```python
from build123d import *
from OCP.BRepFilletAPI import BRepFilletAPI_MakeChamfer

# Parameters (mm, degrees)
SKETCH_1_W           = 177
SKETCH_1_H           = 15
EXTRUDE_1_DEPTH      = 5
SKETCH_3_W           = 15
SKETCH_3_H           = 55
EXTRUDE_3_DEPTH      = 5
SKETCH_9_W           = 33
SKETCH_9_H           = 35
EXTRUDE_5_DEPTH      = 5
CUT_EXTRUDE_4_REACH  = 115.989
CUT_EXTRUDE_5_REACH  = 115.989
SKETCH_10_R          = 3
SKETCH_13_W          = 28
SKETCH_13_H          = 25
CUT_EXTRUDE_8_DEPTH  = 10
CHAMFER_4_SIZE       = 5
FILLET_3_R           = 3
SKETCH_14_W          = 6
SKETCH_14_H          = 11
CUT_EXTRUDE_9_DEPTH  = 10
SKETCH_15_R          = 3.5
CUT_EXTRUDE_10_DEPTH = 10
CHAMFER_5_SIZE       = 2
CHAMFER_5_SIZE2      = 2.22122503


with BuildPart() as part:
    # 스케치1 → 보스-돌출1 (new body)
    with BuildSketch(Plane.XY):
        Rectangle(SKETCH_1_W, SKETCH_1_H)
    extrude(amount=EXTRUDE_1_DEPTH)

    # 스케치3 → 보스-돌출3 (add)
    with BuildSketch(Plane.XY.offset(5)):
        with Locations((96, -20)):
            Rectangle(SKETCH_3_W, SKETCH_3_H)
        with Locations((-96, -20)):
            Rectangle(SKETCH_3_W, SKETCH_3_H)
    extrude(amount=-EXTRUDE_3_DEPTH)

    # 스케치9 → 보스-돌출5 (add)
    with BuildSketch(Plane.XY.offset(5)):
        with Locations((-72, -30)):
            Rectangle(SKETCH_9_W, SKETCH_9_H)
        with Locations((72, -30)):
            Rectangle(SKETCH_9_W, SKETCH_9_H)
    extrude(amount=-EXTRUDE_5_DEPTH)

    # 스케치8 → 컷-돌출4 (cut, up to next)
    with BuildSketch(Plane.XY.offset(5), mode=Mode.PRIVATE) as cut_extrude_4_sk1:
        with BuildLine():
            Line((-88.5, -7.5), (-88.7, -7.5))
            ThreePointArc((-88.7, -7.5), (-89.407106781, -7.792893219), (-89.7, -8.5))
            Line((-89.7, -8.5), (-89.7, -11.5))
            ThreePointArc((-89.7, -11.5), (-89.407106781, -12.207106781), (-88.7, -12.5))
            Line((-88.7, -12.5), (-88.5, -12.5))
            Line((-88.5, -12.5), (-88.5, -7.5))
        make_face()
    cut_extrude_4_tool1 = extrude(cut_extrude_4_sk1.sketch, amount=-CUT_EXTRUDE_4_REACH, mode=Mode.PRIVATE) & part.part
    # 스케치8 → 컷-돌출4 (cut, up to next)
    with BuildSketch(Plane.XY.offset(5), mode=Mode.PRIVATE) as cut_extrude_4_sk2:
        with BuildLine():
            Line((88.5, -7.5), (88.7, -7.5))
            ThreePointArc((88.7, -7.5), (89.407106781, -7.792893219), (89.7, -8.5))
            Line((89.7, -8.5), (89.7, -11.5))
            ThreePointArc((89.7, -11.5), (89.407106781, -12.207106781), (88.7, -12.5))
            Line((88.7, -12.5), (88.5, -12.5))
            Line((88.5, -12.5), (88.5, -7.5))
        make_face()
    cut_extrude_4_tool2 = extrude(cut_extrude_4_sk2.sketch, amount=-CUT_EXTRUDE_4_REACH, mode=Mode.PRIVATE) & part.part
    add(cut_extrude_4_tool1.solids().sort_by_distance((-89.070982, -10, 5))[0], mode=Mode.SUBTRACT)
    add(cut_extrude_4_tool2.solids().sort_by_distance((89.070982, -10, 5))[0], mode=Mode.SUBTRACT)

    # 스케치10 → 컷-돌출5 (cut, up to next)
    with BuildSketch(Plane.XY.offset(5), mode=Mode.PRIVATE) as cut_extrude_5_sk1:
        with Locations((65, -36.5)):
            Circle(SKETCH_10_R)
    cut_extrude_5_tool1 = extrude(cut_extrude_5_sk1.sketch, amount=-CUT_EXTRUDE_5_REACH, mode=Mode.PRIVATE) & part.part
    # 스케치10 → 컷-돌출5 (cut, up to next)
    with BuildSketch(Plane.XY.offset(5), mode=Mode.PRIVATE) as cut_extrude_5_sk2:
        with Locations((-65, -36.5)):
            Circle(SKETCH_10_R)
    cut_extrude_5_tool2 = extrude(cut_extrude_5_sk2.sketch, amount=-CUT_EXTRUDE_5_REACH, mode=Mode.PRIVATE) & part.part
    add(cut_extrude_5_tool1.solids().sort_by_distance((65, -36.5, 5))[0], mode=Mode.SUBTRACT)
    add(cut_extrude_5_tool2.solids().sort_by_distance((-65, -36.5, 5))[0], mode=Mode.SUBTRACT)

    # 스케치13 → 컷-돌출8 (cut)
    with BuildSketch(Plane(origin=(0, 0, 0), x_dir=(-1, 0, 0), z_dir=(0, 0, -1))):
        with Locations((-89.5, -35)):
            Rectangle(SKETCH_13_W, SKETCH_13_H)
        with Locations((89.5, -35)):
            Rectangle(SKETCH_13_W, SKETCH_13_H)
    extrude(amount=-CUT_EXTRUDE_8_DEPTH, mode=Mode.SUBTRACT)

    # 모따기4
    chamfer_4_edges = [part.edges().sort_by_distance(p)[0] for p in [
        (103.5, -22.5, 2.5),
        (-103.5, -22.5, 2.5),
        (103.5, 7.5, 2.5),
        (-103.5, 7.5, 2.5),
        (-55.5, -12.5, 2.5),
        (55.5, -12.5, 2.5),
    ]]
    chamfer(chamfer_4_edges, length=CHAMFER_4_SIZE)

    # 필렛3
    fillet_3_edges = [part.edges().sort_by_distance(p)[0] for p in [
        (75.5, -22.5, 2.5),
        (-75.5, -22.5, 2.5),
    ]]
    fillet(fillet_3_edges, radius=FILLET_3_R)

    # 스케치14 → 컷-돌출9 (cut)
    with BuildSketch(Plane(origin=(0, 0, 0), x_dir=(-1, 0, 0), z_dir=(0, 0, -1))):
        with Locations((-65, -42)):
            Rectangle(SKETCH_14_W, SKETCH_14_H)
        with Locations((65, -42)):
            Rectangle(SKETCH_14_W, SKETCH_14_H)
    extrude(amount=-CUT_EXTRUDE_9_DEPTH, mode=Mode.SUBTRACT)

    # 스케치15 → 컷-돌출10 (cut)
    with BuildSketch(Plane(origin=(0, 0, 0), x_dir=(-1, 0, 0), z_dir=(0, 0, -1))):
        with Locations((65, -36.5)):
            Circle(SKETCH_15_R)
        with Locations((-65, -36.5)):
            Circle(SKETCH_15_R)
    extrude(amount=-CUT_EXTRUDE_10_DEPTH, mode=Mode.SUBTRACT)

    # 모따기5: one chamfer whose edges measure the first distance from different faces: ONE call of the kernel's chamfer builder (chamfer() names one face for all edges)
    chamfer_5_edges_1 = [part.edges().sort_by_distance(p)[0] for p in [
        (75.5, -47.5, 2.5),
    ]]
    chamfer_5_side_1 = [part.faces().sort_by_distance(p)[0] for p in [
        (71.75, -47.5, 2.5),
    ]]
    chamfer_5_edges_2 = [part.edges().sort_by_distance(p)[0] for p in [
        (-75.5, -47.5, 2.5),
    ]]
    chamfer_5_side_2 = [part.faces().sort_by_distance(p)[0] for p in [
        (-75.5, -36.5, 2.5),
    ]]
    chamfer_5_edges_3 = [part.edges().sort_by_distance(p)[0] for p in [
        (-55.5, -47.5, 2.5),
    ]]
    chamfer_5_side_3 = [part.faces().sort_by_distance(p)[0] for p in [
        (-55.5, -32.5, 2.5),
    ]]
    chamfer_5_edges_4 = [part.edges().sort_by_distance(p)[0] for p in [
        (55.5, -47.5, 2.5),
    ]]
    chamfer_5_side_4 = [part.faces().sort_by_distance(p)[0] for p in [
        (58.75, -47.5, 2.5),
    ]]
    chamfer_5 = BRepFilletAPI_MakeChamfer(part.part.solid().wrapped)
    for e in chamfer_5_edges_1:
        chamfer_5.Add(CHAMFER_5_SIZE, CHAMFER_5_SIZE2, e.wrapped, chamfer_5_side_1[0].wrapped)  # the first distance lies on this face
    for e in chamfer_5_edges_2:
        chamfer_5.Add(CHAMFER_5_SIZE, CHAMFER_5_SIZE2, e.wrapped, chamfer_5_side_2[0].wrapped)  # the first distance lies on this face
    for e in chamfer_5_edges_3:
        chamfer_5.Add(CHAMFER_5_SIZE, CHAMFER_5_SIZE2, e.wrapped, chamfer_5_side_3[0].wrapped)  # the first distance lies on this face
    for e in chamfer_5_edges_4:
        chamfer_5.Add(CHAMFER_5_SIZE, CHAMFER_5_SIZE2, e.wrapped, chamfer_5_side_4[0].wrapped)  # the first distance lies on this face
    add(Compound.cast(chamfer_5.Shape()), mode=Mode.REPLACE)


solid = part.part
```
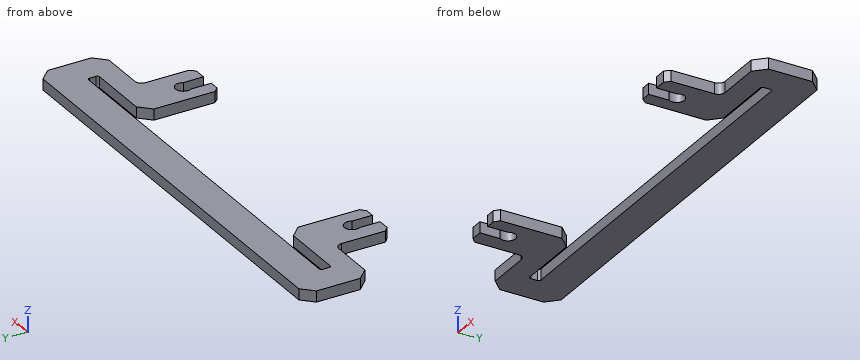
Verification items for the finished model (mm, model axes). Round coordinates to 2 decimals unless told otherwise and drop trailing zeros. Write each loop counter-clockwise with the first axis right and the second up, starting at its lowest first coordinate (ties: lowest second). Pieces come first, ordered by that corner, then holes. Notation, with made-up numbers: (34.5, 11.25) -> (61.5, 11.25) arc R32 cw to (61.5, 44.25) -> close; hole circle Ø8 at (89, 65). An arc over 180 degrees is marked (long way). Write each question's results on one line, items separated by ' | '. Start each with the question number.
1. Cross-section at B-B (y = -36.5). Enter the section's corners in (x, z).
2. Cross-section at D-D (x = -2.5). Enter the section's corners in (y, z), then the cut area to 3 significant figures.
3. Material ranges on probe 1 along X at (y, z) = (-36, 2.1); probe 2 along X at (y, z) = (-29.5, 3.25); probe 3 along Y at (x, z) = (78, 0.7), recorded low to high. Write a range as from..to.
4. Cross-section at A-A (x = -65). Enter the section's corners in (y, z), then the cut area to 4 significant figures.
5. Cross-section at C-C (y = -20.5). Enter the section's corners in (x, z), then the cut area to 3 significant figures.
6. Depth check by flat-ended pin: P1, Ø5.5, axis at x = -65, y = -36.5, coming from the +Z side; P2, Ø2.5, axis at y = -31.5, z = 3.5, coming from the -X side; P3, Ø2.5, axis at y = -38.5, z = 3, coming from the +X side. Enter the tip coordinate at first touch or a pass-through.
Solutions:
1) outline: (-75.5, 0) -> (-68.5, 0) -> (-68.5, 5) -> (-75.5, 5) -> close; (-61.5, 0) -> (-55.5, 0) -> (-55.5, 5) -> (-61.5, 5) -> close; (55.5, 0) -> (61.5, 0) -> (61.5, 5) -> (55.5, 5) -> close; (68.5, 0) -> (75.5, 0) -> (75.5, 5) -> (68.5, 5) -> close
2) outline: (-7.5, 0) -> (7.5, 0) -> (7.5, 5) -> (-7.5, 5) -> close | area: 75.0 mm2
3) probe 1: x = -75.5..-68.46, -61.54..-55.5, 55.5..61.54, 68.46..75.5 | probe 2: x = -75.5..-55.5, 55.5..75.5 | probe 3: y = -22.54..-12.5, -7.5..7.5
4) outline: (-33, 0) -> (-12.5, 0) -> (-12.5, 5) -> (-33, 5) -> close; (-7.5, 0) -> (7.5, 0) -> (7.5, 5) -> (-7.5, 5) -> close | area: 177.5 mm2
5) outline: (-100.5, 0) -> (-55.5, 0) -> (-55.5, 5) -> (-100.5, 5) -> close; (55.5, 0) -> (100.5, 0) -> (100.5, 5) -> (55.5, 5) -> close | area: 450 mm2
6) P1: passes through | P2: stops at x = -75.5 | P3: stops at x = 75.5
